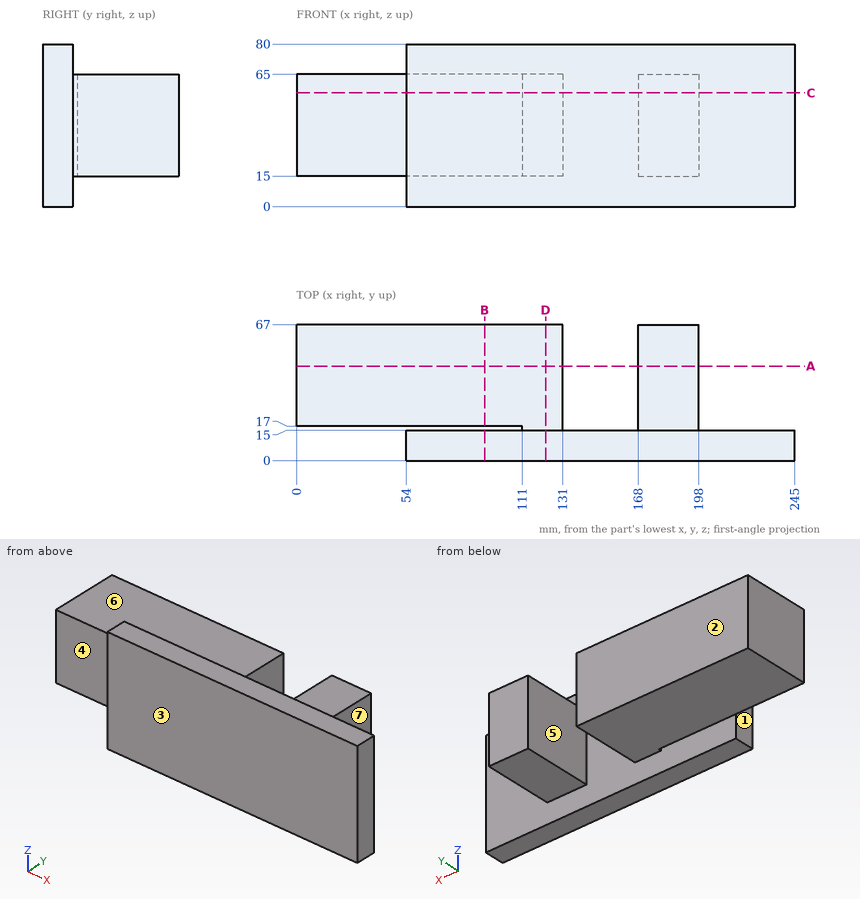
Part print with two shaded views. Sizes in mm from the minimum x, y, z corner. A direction names the side the tool comes from. Give positions to 0.01 mm unless a question says otherwise; leave off trailing zeros. Loops run counter-clockwise (first coordinate to the right, second up) from the corner with the lowest first, then second, coordinate; pieces in that order, holes last. Notation, with made-up numbers: (-40, 72.5) - (-18, 72.5) arc R12 cw to (-18, 94.5) - close; hole circle Ø1 at (16, -24.5). An arc over 180 degrees is marked (long way). Put each result on its own line as item: value.
Q1. Mould opens along Y. For the marked faces 1, 2, 3 and 4 say: pulls with the +Y half, pulls with the -Y half, needs draft (parallel to the pull), parting line crosses it, or undercut.
Filled in:
face 1: needs draft
face 2: pulls with the +Y half
face 3: pulls with the -Y half
face 4: undercut
Q2. Probe line 1 along X through (y, z) = (54, 27.5); line 2 along Z through (x, y) = (49, 23); line 3 along Y through (x, z) = (34, 62.5). List the from-to ranges inside material, lowest first.
Filled in:
line 1: x = 0 to 131, 168 to 198
line 2: z = 15 to 65
line 3: y = 17 to 67
Q3. Slice it at C-C (z = 56). Give the cut face in (x, y).
Filled in:
outline: (0, 17) - (111, 17) - (111, 15) - (54, 15) - (54, 0) - (245, 0) - (245, 15) - (198, 15) - (198, 67) - (168, 67) - (168, 15) - (131, 15) - (131, 67) - (0, 67) - close
Q4. Flat gauge pins, fed straight in: pin 1 (1 mm diameter, centred on x = 76.5, z = 8.5, fed in from +Y); pin 2 (7.5 mm diameter, centred on y = 7.5, z = 50.5, fed in from -X); pin 3 (2 mm diameter, centred on x = 30.5, y = 28, fed in from -Z). Where does each tip first touch, or does it go through?
Filled in:
pin 1: stops at y = 15
pin 2: stops at x = 54
pin 3: stops at z = 15
Q5. Slice it at A-A (y = 46.5). Give the cut face in (x, z), plus the area to 3 significant figures.
Filled in:
outline: (0, 15) - (131, 15) - (131, 65) - (0, 65) - close; (168, 15) - (198, 15) - (198, 65) - (168, 65) - close
area: 8,050 mm²
Q6. Slice it at D-D (x = 122.5). Give the cut face in (y, z).
Filled in:
outline: (0, 0) - (15, 0) - (15, 15) - (67, 15) - (67, 65) - (15, 65) - (15, 80) - (0, 80) - close
Q7. Slice it at B-B (x = 92.5). Give the cut face in (y, z), plus the area to 3 significant figures.
Filled in:
outline: (0, 0) - (15, 0) - (15, 80) - (0, 80) - close; (17, 15) - (67, 15) - (67, 65) - (17, 65) - close
area: 3,700 mm²
Q8. Tool access for the marked faces 5, 6 and 7: list every direction of +Z, -Z, +X, -X, +Y, -Y with a clear straight run to the whole face (end or side of a thin tool).
Filled in:
face 5: +Z, -Z, +Y
face 6: +Z, +X, -X, +Y
face 7: +Z, -Z, +X, +Y
